```python
from build123d import *

# Parameters (mm, degrees)
SKETCH1_R           = 3.175
BOSS_EXTRUDE1_DEPTH = 146.05
BOSS_EXTRUDE2_DEPTH = 3.175
SKETCH3_W           = 58.42
SKETCH3_H           = 9.525
BOSS_EXTRUDE3_DEPTH = 3.175


with BuildPart() as part:
    # Sketch1 → Boss-Extrude1 (new body)
    with BuildSketch(Plane.XY):
        with BuildLine():
            Line((40.420068278, 3.055455197), (32.800068278, -3.294544803))
            Line((32.800068278, -3.294544803), (-17.999931722, -3.294544803))
            ThreePointArc((-17.999931722, -3.294544803), (-29.849193037, -0.119544803), (-17.999931722, 3.055455197))
            Line((-17.999931722, 3.055455197), (40.420068278, 3.055455197))
        make_face()
        with Locations((-23.499193037, -0.119544803)):
            Circle(SKETCH1_R, mode=Mode.SUBTRACT)
    extrude(amount=BOSS_EXTRUDE1_DEPTH)

    # Sketch2 → Boss-Extrude2 (add)
    with BuildSketch(Plane.XY.offset(3.175)):
        Polygon((-17.999931722, 3.055455197), (-14.824931722, 3.055455197), (-14.824931722, 9.405455197), (37.245068278, 9.405455197), (37.245068278, 3.055455197), (40.420068278, 3.055455197), (40.420068278, 12.580455197), (-17.999931722, 12.580455197), align=None)
    extrude(amount=BOSS_EXTRUDE2_DEPTH)

    # Sketch3 → Boss-Extrude3 (add)
    with BuildSketch(Plane.XY.offset(6.35)):
        with Locations((11.210068278, 7.817955197)):
            Rectangle(SKETCH3_W, SKETCH3_H)
    extrude(amount=BOSS_EXTRUDE3_DEPTH)


solid = part.part
```
The model under review builds one solid part; all positions refer to its coordinate system, in mm. A direction names the side the tool comes from. Round coordinates to 2 decimals unless told otherwise and drop trailing zeros. Write each loop counter-clockwise with the first axis right and the second up, starting at its lowest first coordinate (ties: lowest second). Pieces come first, ordered by that corner, then holes.
(1) Mouldability with a two-part tool opening along X and no side actions: class faces 1 (the flat face through (6, 0, 0)), 2 (the flat face through (36.66, -0.08, 72)), 3 (the cylindrical face through (-20.47, 0.83, 72)) as +X half, -X half, draft (parallel to the pull), parting line (faces both ways), or undercut.
(2) Insertion check: pin 1 (7.5 mm diameter, centred on x = 7.5, y = 10, fed in from -Z) (3 decimals); pin 2 (6 mm diameter, centred on y = -3.5, z = 90, fed in from -X); pin 3 (3 mm diameter, centred on x = -2, z = 34, fed in from +Y); pin 4 (2 mm diameter, centred on y = 7.5, z = 52.5, fed in from -X). Each pin has a flat end and moves straight along its axis. Give the tip position at first contact, or say it passes through.
(3) Wall thickness on L1, parallel to Y at x = 12, z = 6; L2, parallel to Y at x = -16, z = 88.5; L3, parallel to X at y = 0.5, z = 104.5: over which ranges is each line inside the solid? List them lowest first.
(4) Machinability: for faces 4 (the flat face through (11, 8, 9.525)), 5 (the flat face through (8, -3.295, 72)), 6 (the flat face through (11, 3.055, 3)), 7 (the flat face through (11, 12.58, 6)), which of the approach directions +Z, -Z, +X, -X, +Y, -Y give a long, thin tool a straight path to every point of the face, cutting with its end or side? Answer none if there is none.
(5) We need section C-C on x = 34.5. Give the boundary of the cut face in (y, z) (3 decimals), and give its area (3 significant figures).
(6) We need section A-A on x = 4. Give the boundary of the cut face in (y, z) (3 decimals).
(7) We need section B-B on z = 20. Give the boundary of the cut face in (x, y) (3 decimals), and give its area (3 significant figures).
Findings below:
1. face 1: draft
1. face 2: +X half
1. face 3: undercut
2. pin 1: stops at z = 3.175
2. pin 2: stops at x = -29.84
2. pin 3: stops at y = 3.06
2. pin 4: passes through
3. L1: y = -3.29 to 3.06, 9.41 to 12.58
3. L2: y = -3.29 to 3.06
3. L3: x = -29.82 to -26.61, -20.39 to 37.35
4. face 4: +Z, +X, +Y
4. face 5: +Z, -Z, +X, -Y
4. face 6: -Z
4. face 7: +Z, -Z, +X, -X, +Y
5. outline: (-1.878, 0) - (3.055, 0) - (3.055, 6.35) - (9.405, 6.35) - (9.405, 3.175) - (12.58, 3.175) - (12.58, 9.525) - (3.055, 9.525) - (3.055, 146.05) - (-1.878, 146.05) - close
5. area: 761 mm2
6. outline: (-3.295, 0) - (3.055, 0) - (3.055, 6.35) - (9.405, 6.35) - (9.405, 3.175) - (12.58, 3.175) - (12.58, 9.525) - (3.055, 9.525) - (3.055, 146.05) - (-3.295, 146.05) - close
7. outline: (-18, -3.295) - (32.8, -3.295) - (40.42, 3.055) - (-18, 3.055) arc R6.35 ccw (long way) to start; hole circle Ø6.35 at (-23.499, -0.12)
7. area: 438 mm2
